Can you work these out from the model? Positions are in its coordinate system, mm. A direction names the side the tool comes from. Give positions to 0.01 mm unless a question says otherwise; leave off trailing zeros. Write each loop counter-clockwise with the first axis right and the second up, starting at its lowest first coordinate (ties: lowest second). Pieces come first, ordered by that corner, then holes. Notation, with made-up numbers: (31.5, 15) - (64.5, 15) arc R18 ccw to (64.5, 35) - close; hole circle Ø11 at (-21, 73). An arc over 180 degrees is marked (long way). Return JSON: item names as keys, results as strings. Group by question number.
from build123d import *

# Parameters (mm, degrees)
SKETCH_1_W          = 12.1
SKETCH_1_H          = 6.1
EXTRUDE_1_DEPTH     = 5
SKETCH_3_R          = 2.5
EXTRUDE_2_DEPTH     = 2
SKETCH_4_R          = 0.75
EXTRUDE_3_DEPTH     = 1
FILLET_1_R          = 0.5
CUT_EXTRUDE_START   = -0.875
CUT_EXTRUDE_2_DEPTH = 0.875
CUT_EXTRUDE_4_DEPTH = 2
FILLET_2_R          = 0.5
SKETCH_10_W         = 1.1
SKETCH_10_H         = 2.146086497
SKETCH_10_W_2       = 2.1
SKETCH_10_H_2       = 0.5
SKETCH_10_W_3       = 0.3
SKETCH_10_H_3       = 1.5
CUT_EXTRUDE_5_DEPTH = 0.875
SKETCH_11_W         = 2.1
SKETCH_11_H         = 0.25
CUT_EXTRUDE_6_DEPTH = 3.25
SKETCH_12_W         = 0.3
SKETCH_12_H         = 1.5
CUT_EXTRUDE_7_DEPTH = 3


with BuildPart() as part:
    # 草图1 → 凸台-拉伸1 (new body)
    with BuildSketch(Plane(origin=(0, 0, 0), x_dir=(1, 0, 0), z_dir=(0, 1, 0))):
        with Locations((6.05, 0)):
            Rectangle(SKETCH_1_W, SKETCH_1_H)
    extrude(amount=EXTRUDE_1_DEPTH)

    # 草图3 → 凸台-拉伸2 (add)
    with BuildSketch(Plane.ZY):
        with Locations((0, 2.5)):
            Circle(SKETCH_3_R)
    extrude(amount=EXTRUDE_2_DEPTH)

    # 草图4 → 凸台-拉伸3 (add)
    with BuildSketch(Plane.XZ):
        with Locations((1.6, 0)):
            Circle(SKETCH_4_R)
        with Locations((8.6, 0)):
            Circle(SKETCH_4_R)
    extrude(amount=EXTRUDE_3_DEPTH)

    # 圆角1
    fillet_1_edges = [part.edges().sort_by_distance(p)[0] for p in [
        (0.85, -1, 0),
        (7.85, -1, 0),
    ]]
    fillet(fillet_1_edges, radius=FILLET_1_R)

    # 草图6 → 切除-拉伸2 (cut)
    with BuildSketch(Plane(origin=(0, 0, -3.05), x_dir=(-1, 0, 0), z_dir=(0, 0, -1)).offset(CUT_EXTRUDE_START)):
        Polygon((-1.75, 0), (-1.75, 3.5), (-2.615259451, 3.5), (-2.615259451, 0.5), (-3.7, 0.5), (-3.7, 0), align=None)
        Polygon((-6.7, 0.5), (-6.7, 0), (-4.75, 0), (-4.75, 3.5), (-5.615259451, 3.5), (-5.615259451, 0.5), align=None)
        Polygon((-8.75, 3.5), (-9.615259451, 3.5), (-9.615259451, 0.5), (-10.7, 0.5), (-10.7, 0), (-8.75, 0), align=None)
    extrude(amount=CUT_EXTRUDE_2_DEPTH, mode=Mode.SUBTRACT)

    # 草图8 → 切除-拉伸4 (cut)
    with BuildSketch(Plane(origin=(0, 5, 0), x_dir=(1, 0, 0), z_dir=(0, 1, 0))):
        Polygon((8.35, 2.55), (11.1, 2.55), (11.1, 2.290157714), (10.8, 2.290157714), (10.8, 0.35), (8.65, 0.35), (8.65, 2.290157714), (8.35, 2.290157714), align=None)
        Polygon((4.35, 2.55), (7.1, 2.55), (7.1, 2.290157714), (6.8, 2.290157714), (6.8, 0.35), (4.65, 0.35), (4.65, 2.290157714), (4.35, 2.290157714), align=None)
        Polygon((1.35, 2.55), (4.1, 2.55), (4.1, 2.290157714), (3.8, 2.290157714), (3.8, 0.35), (1.65, 0.35), (1.65, 2.290157714), (1.35, 2.290157714), align=None)
    extrude(amount=-CUT_EXTRUDE_4_DEPTH, mode=Mode.SUBTRACT)

    # 草图9 → 切除-旋转1 (revolve, cut)
    with BuildSketch(Plane(origin=(0, 2.5, 0), x_dir=(1, 0, 0), z_dir=(0, 1, 0))):
        Polygon((-2, 0), (-2, 1.8), (5, 1.8), (5, 1.5), (8, 1.5), (8, 1.25), (12.1, 1.25), (12.1, 0), align=None)
    revolve(axis=Axis((-0.907835796, 2.5, 0), (1, 0, 0)), mode=Mode.SUBTRACT)

    # 圆角2
    fillet_2_edges = [part.edges().sort_by_distance(p)[0] for p in [
        (-2, 2.5, -2.5),
    ]]
    fillet(fillet_2_edges, radius=FILLET_2_R)

    # 草图10 → 切除-拉伸5 (cut)
    with BuildSketch(Plane.XY.offset(3.05).offset(CUT_EXTRUDE_START)):
        with Locations((10.55, 3.926956752)):
            Rectangle(SKETCH_10_W, SKETCH_10_H)
        with Locations((11.05, 0.25)):
            Rectangle(SKETCH_10_W_2, SKETCH_10_H_2)
        with Locations((11.95, 2.5)):
            Rectangle(SKETCH_10_W_3, SKETCH_10_H_3)
    extrude(amount=CUT_EXTRUDE_5_DEPTH, mode=Mode.SUBTRACT)

    # 草图11 → 切除-拉伸6 (cut)
    with BuildSketch(Plane.XZ):
        with Locations((11.05, 2.3)):
            Rectangle(SKETCH_11_W, SKETCH_11_H)
    extrude(amount=-CUT_EXTRUDE_6_DEPTH, mode=Mode.SUBTRACT)

    # 草图12 → 切除-拉伸7 (cut)
    with BuildSketch(Plane.XY.offset(3.05)):
        with Locations((11.95, 2.5)):
            Rectangle(SKETCH_12_W, SKETCH_12_H)
    extrude(amount=-CUT_EXTRUDE_7_DEPTH, mode=Mode.SUBTRACT)


solid = part.part
1) Imagine slicing it at B-B, the plane x = -0.75. Write out the boundary of the cut face in (y, z).
2) Imagine slicing it at C-C, the plane z = -0.5. Count the separate pieces of the cut face and the enclosed holes in it, and give its area (3 significant figures).
3) Will these pins go through, and if not, where does the flat tip stop? pin 1 Ø0.6 at (y, z) = (2.5, 1.5) entering from +X; pin 2 Ø3 at (x, z) = (4, 1) entering from -Y; pin 3 Ø0.9 at (y, z) = (2, -0.5) entering from -X.
4) We'd pull the mould along X, two halves only. Please class faces 1 (the face through (11, 2, 2.425)), 2 (the face through (9.615, 2, -2.6)), 3 (the face through (12.1, 3.02, -1.31)): pulls with the +X half, pulls with the -X half, needs draft (parallel to the pull), parting line crosses it, or undercut.
5) I need wall thicknesses on line 1 along Z through (x, y) = (11.25, 3.5); line 2 along Z through (x, y) = (5.7, 2.5); line 3 along Y through (x, z) = (11.75, 0). Which ranges of each line are inside material? Lowest first, please.
6) Imagine slicing it at A-A, the plane x = 3.5. Write out the boundary of the cut face in (y, z) (3 decimals), and give its area (3 significant figures).
7) On a 3-axis mill with a long thin cutter (end or side, diameter ignored), from which of +Z, -Z, +X, -X, +Y, -Y can I reach the whole of each face in a straight line? I mean faces 4 (the face through (7, 1, 0)), 5 (the face through (6, 4, -2.55)), 6 (the face through (11.8, 2, 2)). Say none if no direction works.
Resolved:
{
 "1": {"outline": "circle Ø5 at (2.5, 0); hole circle Ø3.6 at (2.5, 0)"},
 "2": {"separate pieces": "5", "enclosed holes": "0", "area": "23.2 mm^2"},
 "3": {"pin 1": "x = 11.8", "pin 2": "y = 0", "pin 3": "through"},
 "4": {"face 1": "needs draft", "face 2": "undercut", "face 3": "pulls with the +X half"},
 "5": {"line 1": "-3.05 to -0.75, 0.75 to 3.05", "line 2": "-3.05 to -1.5, 1.5 to 3.05", "line 3": "0 to 1.25, 3.75 to 5"},
 "6": {"outline": "(0, -2.175) - (0.5, -2.175) - (0.5, -3.05) - (5, -3.05) - (5, -2.55) - (3, -2.55) - (3, -1.729) arc R1.8 cw (long way) to (4.266, -0.35) - (5, -0.35) - (5, 3.05) - (0, 3.05) - close", "area": "16.7 mm^2"},
 "7": {"face 4": "-X", "face 5": "+Y", "face 6": "+Z, +X"}
}
